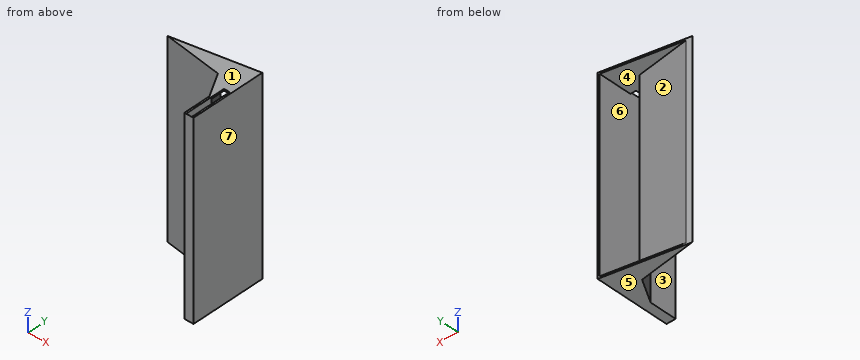
```python
from build123d import *

# Parameters (mm, degrees)
BOSS_EXTRUDE1_DEPTH = 701.675
SHELL1_T            = -12.7
SKETCH3_W           = 42
SKETCH3_H           = 290
CUT_EXTRUDE1_DEPTH  = 20
BOSS_EXTRUDE2_REACH = 957.285
CHAMFER1_SIZE       = 12.7
CHAMFER1_SIZE_2     = 20


with BuildPart() as part:
    # Sketch2 → Boss-Extrude1 (new, symmetric)
    with BuildSketch(Plane.XY):
        Polygon((0, 0), (-105, 181.865334795), (-532.938806236, 244.144070894), (67.4, 350), (67.4, -200), (0, -200), align=None)
    extrude(amount=BOSS_EXTRUDE1_DEPTH, both=True)

    # Shell1
    shell1_openings = [part.faces().sort_by_distance(p)[0] for p in [
        (-232.769403118, 297.072035447, 0),
    ]]
    offset(amount=SHELL1_T, openings=shell1_openings, kind=Kind.INTERSECTION)

    # Sketch3 → Cut-Extrude1 (cut)
    with BuildSketch(Plane.XY.offset(701.675)):
        with Locations((33.7, -42.3)):
            Rectangle(SKETCH3_W, SKETCH3_H)
    extrude(amount=-CUT_EXTRUDE1_DEPTH, mode=Mode.SUBTRACT)

    # Sketch4 → Boss-Extrude2 (add, up to next)
    with BuildSketch(Plane(origin=(12.7, 0, 0), x_dir=(0, 0, -1), z_dir=(1, 0, 0)), mode=Mode.PRIVATE) as boss_extrude2_sk1:
        Polygon((688.975, -187.3), (688.975, -67.383663338), (-681.675, -187.3), align=None)
    boss_extrude2_tool1 = extrude(boss_extrude2_sk1.sketch, amount=BOSS_EXTRUDE2_REACH, mode=Mode.PRIVATE) - part.part
    add(boss_extrude2_tool1.solids().sort_by_distance((12.7, -147.327888, -232.091667))[0])

    # Chamfer1
    # the kernel refuses this chamfer: 20, 12.7 mm, written as the material it adds along each edge
    # the kernel refuses this chamfer: 20, 12.7 mm, written as the material it takes off along each edge
    with BuildSketch(Plane(origin=(12.7, -187.3, 701.675), x_dir=(0, -0.9986795899881412, 0.05137194313161755), z_dir=(1, 0, 0))) as chamfer1_2_piece_1:
        Polygon((CHAMFER1_SIZE * 0.998679589988, CHAMFER1_SIZE * 0.0513719431316), (-CHAMFER1_SIZE_2 * 0.0513719431316, CHAMFER1_SIZE_2 * 0.998679589988), (0, 0), align=None)
    extrude(amount=42, mode=Mode.SUBTRACT)


solid = part.part
```
Can you work these out from the model? Positions are in its coordinate system, mm. Face numbers are marked on the shaded views. A direction names the side the tool comes from. Give positions to 0.01 mm unless a question says otherwise; leave off trailing zeros. Write each loop counter-clockwise with the first axis right and the second up, starting at its lowest first coordinate (ties: lowest second). Pieces come first, ordered by that corner, then holes. Notation, with made-up numbers: (-8, 50) -> (51, 50) arc R11 cw to (51, 61) -> close; hole circle Ø11 at (-27, 31.25). An arc over 180 degrees is marked (long way). One line per item, written item: value.
Q1. Imagine slicing it at D-D on z = -167. Please give me the cut outline in (x, y).
Results found:
outline: (-532.94, 244.14) -> (-105, 181.87) -> (0, 0) -> (0, -200) -> (67.4, -200) -> (67.4, 350) -> (54.7, 347.76) -> (54.7, -113.05) -> (12.7, -113.05) -> (12.7, 3.4) -> (-97.08, 193.55) -> (-493.06, 251.17) -> close
Q2. We'd pull the mould along Z, two halves only. Please class the marked faces 4, 5, 6 and 7: +Z half, -Z half, draft (parallel to the pull), parting line (faces both ways), or undercut.
Results found:
face 4: undercut
face 5: -Z half
face 6: undercut
face 7: draft
Q3. Imagine slicing it at A-A on y = -31. Please give me the cut outline in (x, z) (3 decimals).
Results found:
outline: (0, -701.675) -> (67.4, -701.675) -> (67.4, 701.675) -> (54.7, 701.675) -> (54.7, -688.975) -> (12.7, -688.975) -> (12.7, 701.675) -> (0, 701.675) -> close
Q4. Imagine slicing it at C-C on x = -61. Please give me the cut outline in (y, z) (3 decimals).
Results found:
outline: (105.655, -701.675) -> (327.36, -701.675) -> (327.36, -688.975) -> (131.055, -688.975) -> (131.055, 688.975) -> (327.36, 688.975) -> (327.36, 701.675) -> (105.655, 701.675) -> close
Q5. Please list where these lines run through material, in increasing order: line 1 (Z direction, x = -6, y = 322.5) (3 decimals); line 2 (X direction, y = -17, z = 46); line 3 (X direction, y = 137.5, z = 236). Write a range as [from, to].
Results found:
line 1: z = [-701.675, -688.975], [688.975, 701.675]
line 2: x = [0, 12.7], [54.7, 67.4]
line 3: x = [-79.39, -64.72], [54.7, 67.4]
Q6. Which directions (+Z, -Z, +X, -X, +Y, -Y) give clear straight access to the entire face, cutting with the end or side of a thin tool? Please do the marked faces 1, 2 and 3.
Results found:
face 1: +Z, +X, -X, +Y, -Y
face 2: +Y
face 3: +Z, -Z, -X, -Y
Q7. Imagine slicing it at B-B on z = 35. Please give me the cut outline in (x, y), and give its area (3 significant figures).
Results found:
outline: (-532.94, 244.14) -> (-105, 181.87) -> (0, 0) -> (0, -200) -> (67.4, -200) -> (67.4, 350) -> (54.7, 347.76) -> (54.7, -130.72) -> (12.7, -130.72) -> (12.7, 3.4) -> (-97.08, 193.55) -> (-493.06, 251.17) -> close
area: 20,500 mm^2
Q8. For P1, Ø8, axis at x = -465.5, z = 91.5, coming from the -Y side; P2, Ø12, axis at y = -105, z = -468.5, coming from the -X side; P3, Ø1.5, axis at x = -90.5, z = -543.5, coming from the +Y side, each with a flat end and sliding along its axis, tell me the tip position at first contact or that it passes through.
Results found:
P1: stops at y = 233.75
P2: stops at x = 0
P3: stops at y = 183.45
